For this review, take the finished solid that the model builds, in its own axes (mm). Face numbers are marked on the shaded views. A direction names the side the tool comes from. Round coordinates to 2 decimals unless told otherwise and drop trailing zeros. Loops run counter-clockwise (first coordinate to the right, second up) from the corner with the lowest first, then second, coordinate; pieces in that order, holes last.
1. Consider section D-D on y = -5.25. State the section outline as (x, z) points, then the cut area to 3 significant figures.
2. Consider section A-A on x = 0. State the section outline as (y, z) points, then the cut area to 3 significant figures.
3. Clearance check with flat-ended pins moving along their axes: pin 1 Ø1 at (y, z) = (-9.5, 7.5) entering from -X; pin 2 Ø3 at (y, z) = (11.5, 15.5) entering from -X; pin 3 Ø2 at (x, z) = (-12, 14) entering from -Y. State where each tip first meets the part, or that it passes through.
4. Draft analysis for pull direction X (two halves, no side actions). For the marked faces 5, 6 and 7, state which applies: released by +X, released by -X, zero draft, split by the parting line, or undercut.
5. Consider section B-B on y = 0. State the section outline as (x, z) points.
6. Tool access review of the marked faces 1, 2, 3 and 4: name each direction out of +Z, -Z, +X, -X, +Y, -Y from which nothing blocks a thin tool from reaching the whole face with its end or side.
7. To check wall thickness, follow line 1 along Y through (x, z) = (0, 18.1); line 2 along Y through (x, z) = (0, 7.5); line 3 along X through (y, z) = (-12.5, 6.5). State the ranges of each line that lie inside material, in increasing order.
8. Consider section C-C on z = 17.25. State the section outline as (x, y) points, then the cut area to 3 significant figures.
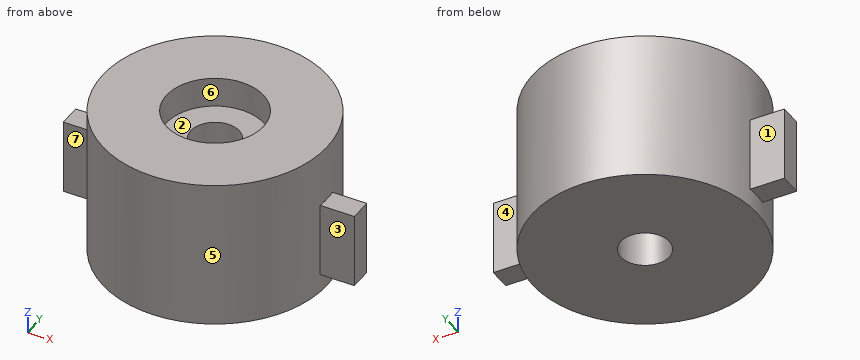
Solid Edge part; units mm, degrees
sketch "Sketch1" plane through (0, 0, 0) normal (0, 0, 1) x (1, 0, 0)
  circle A0 centre (0, 0) radius 15
extrude "Protrusion1" add sketch "Sketch1" along normal blind 20
sketch "Sketch2" plane through (0, 0, 20) normal (0, 0, 1) x (1, 0, 0)
  circle A0 centre (0, 0) radius 3.25
extrude "Cutout1" cut sketch "Sketch2" against normal through all
sketch "Sketch3" plane through (19.5, 0, 0) normal (1, 0, 0) x (0, 1, 0)
  line L0 (-1.5, 2.5) -> (1.5, 2.5)
  line L1 (1.5, 2.5) -> (1.5, 12.5)
  line L2 (1.5, 12.5) -> (-1.5, 12.5)
  line L3 (-1.5, 12.5) -> (-1.5, 2.5)
  dimension "D1" = 1.5
  dimension "D2" = 1.5
extrude "Appoggio_laterale_Profile_Plane1" add sketch "Sketch3" against normal up to next
mirror "Mirror1" about plane through (0, 0, 0) normal (1, 0, 0) of "Appoggio_laterale_Profile_Plane1"
sketch "Sketch4" plane through (0, 0, 20) normal (0, 0, 1) x (1, 0, 0)
  circle A0 centre (0, 0) radius 6.5
extrude "ScavoEstrusione_2" cut sketch "Sketch4" against normal blind 4
Resolved:
1. outline: (-14.05, 0) - (14.05, 0) - (14.05, 20) - (3.83, 20) - (3.83, 16) - (-3.83, 16) - (-3.83, 20) - (-14.05, 20) - close
1. area: 531 mm2
2. outline: (-15, 0) - (-3.25, 0) - (-3.25, 16) - (-6.5, 16) - (-6.5, 20) - (-15, 20) - close; (3.25, 0) - (15, 0) - (15, 20) - (6.5, 20) - (6.5, 16) - (3.25, 16) - close
2. area: 444 mm2
3. pin 1: stops at x = -12
3. pin 2: stops at x = -11.18
3. pin 3: stops at y = -10.2
4. face 5: split by the parting line
4. face 6: undercut
4. face 7: zero draft
5. outline: (-19.5, 2.5) - (-15, 2.5) - (-15, 0) - (-3.25, 0) - (-3.25, 16) - (-6.5, 16) - (-6.5, 20) - (-15, 20) - (-15, 12.5) - (-19.5, 12.5) - close; (3.25, 0) - (15, 0) - (15, 2.5) - (19.5, 2.5) - (19.5, 12.5) - (15, 12.5) - (15, 20) - (6.5, 20) - (6.5, 16) - (3.25, 16) - close
6. face 1: +Z, -Z, -X, +Y
6. face 2: +Z
6. face 3: +Z, -Z, +X, -Y
6. face 4: +Z, -Z, +X, +Y
7. line 1: y = -15 to -6.5, 6.5 to 15
7. line 2: y = -15 to -3.25, 3.25 to 15
7. line 3: x = -8.29 to 8.29
8. outline: circle Ø30 at (0, 0); hole circle Ø13 at (0, 0)
8. area: 574 mm2
